Autodesk Inventor part; units mm, degrees
ref_plane "YZ Plane" through (0, 0, 0) normal (1, 0, 0) x (0, 1, 0)
ref_plane "XZ Plane" through (0, 0, 0) normal (0, 1, 0) x (-1, 0, 0)
ref_plane "XY Plane" through (0, 0, 0) normal (0, 0, 1) x (1, 0, 0)
sketch "Esquisse1" plane through (0, 0, 0) normal (0, 0, 1) x (1, 0, 0)
  line L0 (-12.5, -10) -> (12.5, -10)
  line L1 (12.5, -10) -> (12.5, 10)
  line L2 (12.5, 10) -> (-12.5, 10)
  line L3 (-12.5, 10) -> (-12.5, -10)
  line L4 (-12.5, -10) -> (12.5, 10) construction
  line L5 (12.5, -10) -> (-12.5, 10) construction
  point P0 (0, 0)
  dimension "d0" = 25
  dimension "d1" = 20
extrude "Extrusion1" add sketch "Esquisse1" along normal blind 7
sketch "Esquisse2" plane through (0, 0, 7) normal (0, 0, 1) x (1, 0, 0)
  line L0 (12.5, -10) -> (12.5, 10)
  line L1 (-12.5, 10) -> (-12.5, -10)
  line L2 (12.5, 10) -> (-12.5, 10)
  line L3 (-12.5, 10) -> (-12.5, 5)
  line L4 (-12.5, 5) -> (12.5, 5)
  line L5 (12.5, 5) -> (12.5, 10)
  point P0 (0, 0)
  point P1 (12.5, 5)
  dimension "d4" = 5
extrude "Extrusion2" add sketch "Esquisse2" along normal blind 3
sketch "Esquisse3" plane through (-12.5, 10, 0) normal (0, 1, 0) x (1, 0, 0)
  line L0 (25, 0) -> (25, -10)
  line L1 (25, -10) -> (24.1, -10)
  line L2 (24.1, -10) -> (24.1, -8)
  line L3 (24.1, -8) -> (25, -8)
  line L4 (25, -8) -> (25, -10)
  line L5 (24.1, -10) -> (21.56, -10)
  line L6 (25, -10) -> (0, -10)
  line L7 (21.56, -10) -> (16.1469, -10)
  line L8 (21.56, -10) -> (20.66, -10)
  line L9 (20.66, -10) -> (20.66, -8)
  line L10 (20.66, -8) -> (21.56, -8)
  line L11 (21.56, -8) -> (21.56, -10)
  line L12 (20.66, -10) -> (18.12, -10)
  line L13 (18.12, -10) -> (17.22, -10)
  line L14 (17.22, -10) -> (17.22, -8)
  line L15 (17.22, -8) -> (18.12, -8)
  line L16 (18.12, -8) -> (18.12, -10)
  line L17 (17.22, -10) -> (14.68, -10)
  line L18 (14.68, -10) -> (13.78, -10)
  line L19 (13.78, -10) -> (13.78, -8)
  line L20 (13.78, -8) -> (14.68, -8)
  line L21 (14.68, -8) -> (14.68, -10)
  line L22 (13.78, -10) -> (11.24, -10)
  line L23 (11.24, -10) -> (10.34, -10)
  line L24 (10.34, -10) -> (10.34, -8)
  line L25 (10.34, -8) -> (11.24, -8)
  line L26 (11.24, -8) -> (11.24, -10)
  line L27 (10.34, -10) -> (7.8, -10)
  line L28 (7.8, -10) -> (6.9, -10)
  line L29 (6.9, -10) -> (6.9, -8)
  line L30 (6.9, -8) -> (7.8, -8)
  line L31 (7.8, -8) -> (7.8, -10)
  line L32 (6.9, -10) -> (4.36, -10)
  line L33 (4.36, -10) -> (3.46, -10)
  line L34 (3.46, -10) -> (3.46, -8)
  line L35 (3.46, -8) -> (4.36, -8)
  line L36 (4.36, -8) -> (4.36, -10)
  line L37 (3.46, -10) -> (0.92, -10)
  line L38 (0.92, -10) -> (0.02, -10)
  line L39 (0.02, -8) -> (0.92, -8)
  line L40 (0.92, -8) -> (0.92, -10)
  line L41 (0, -10) -> (0, -8)
  line L42 (0, -8) -> (0.02, -8)
  point P0 (12.5, 0)
  point P1 (3.46, -10)
  point P2 (4.36, -10)
  point P3 (6.9, -10)
  point P4 (7.8, -10)
  dimension "d7" = 2.54
  dimension "d11" = 0.9
  dimension "d12" = 2
  dimension "d13" = 2.54
  dimension "d14" = 0.9
  dimension "d15" = 2
  dimension "d16" = 2.54
  dimension "d17" = 0.9
  dimension "d18" = 2
  dimension "d19" = 2.54
  dimension "d20" = 0.9
  dimension "d21" = 2
  dimension "d22" = 2.54
  dimension "d23" = 0.9
  dimension "d24" = 2
  dimension "d25" = 2.54
  dimension "d26" = 0.9
  dimension "d27" = 2
  dimension "d28" = 2.54
  dimension "d29" = 0.9
  dimension "d30" = 2
  dimension "d33" = 2
extrude "Extrusion3" add sketch "Esquisse3" along normal blind 4
sketch "Esquisse4" plane through (-12.5, 10, 0) normal (0, 1, 0) x (1, 0, 0)
  line L0 (25, -7) -> (25, -10)
  line L1 (25, -10) -> (24.1, -10)
  line L2 (0, -10) -> (25, -10)
  line L3 (24.1, -10) -> (21.56, -10)
  line L4 (21.56, -10) -> (21.56, -8)
  line L5 (21.56, -8) -> (24.1, -8)
  line L6 (24.1, -8) -> (24.1, -10)
  line L7 (21.56, -10) -> (20.66, -10)
  line L8 (20.66, -10) -> (18.12, -10)
  line L9 (18.12, -10) -> (18.12, -8)
  line L10 (18.12, -8) -> (20.66, -8)
  line L11 (20.66, -8) -> (20.66, -10)
  line L12 (18.12, -10) -> (17.22, -10)
  line L13 (17.22, -10) -> (14.68, -10)
  line L14 (14.68, -10) -> (14.68, -8)
  line L15 (14.68, -8) -> (17.22, -8)
  line L16 (17.22, -8) -> (17.22, -10)
  line L17 (14.68, -10) -> (13.78, -10)
  line L18 (13.78, -10) -> (11.24, -10)
  line L19 (11.24, -10) -> (11.24, -8)
  line L20 (11.24, -8) -> (13.78, -8)
  line L21 (13.78, -8) -> (13.78, -10)
  line L22 (11.24, -10) -> (10.34, -10)
  line L23 (10.34, -10) -> (7.8, -10)
  line L24 (7.8, -10) -> (7.8, -8)
  line L25 (7.8, -8) -> (10.34, -8)
  line L26 (10.34, -8) -> (10.34, -10)
  line L27 (7.8, -10) -> (6.9, -10)
  line L28 (6.9, -10) -> (4.36, -10)
  line L29 (4.36, -10) -> (4.36, -8)
  line L30 (4.36, -8) -> (6.9, -8)
  line L31 (6.9, -8) -> (6.9, -10)
  line L32 (4.36, -10) -> (3.46, -10)
  line L33 (3.46, -10) -> (0.92, -10)
  line L34 (0.92, -10) -> (0.92, -8)
  line L35 (0.92, -8) -> (3.46, -8)
  line L36 (3.46, -8) -> (3.46, -10)
  point P0 (12.5, 0)
  point P1 (3.46, -10)
  point P2 (4.36, -10)
  point P3 (6.9, -10)
  point P4 (7.8, -10)
  dimension "d36" = 0.9
  dimension "d37" = 2.54
  dimension "d38" = 2
  dimension "d39" = 0.9
  dimension "d40" = 2.54
  dimension "d41" = 2
  dimension "d42" = 0.9
  dimension "d43" = 2.54
  dimension "d44" = 2
  dimension "d45" = 0.9
  dimension "d46" = 2.54
  dimension "d47" = 2
  dimension "d48" = 0.9
  dimension "d49" = 2.54
  dimension "d50" = 2
  dimension "d51" = 0.9
  dimension "d52" = 2.54
  dimension "d53" = 2
  dimension "d54" = 0.9
  dimension "d55" = 2.54
  dimension "d56" = 2
extrude "Extrusion4" cut sketch "Esquisse4" along normal through all both and the other way through all
properties part number "Gyroscope MPU6050"
CAD build for the part. Positions are in the model's coordinates, mm. A direction names the side the tool comes from. Give positions to 0.01 mm unless a question says otherwise; leave off trailing zeros. Loops run counter-clockwise (first coordinate to the right, second up) from the corner with the lowest first, then second, coordinate; pieces in that order, holes last. Notation, with made-up numbers: M -18.75,88 L 21.25,88 A27 cw 21.25,116 Z; hole C 44,76 d11. An arc over 180 degrees is marked long. Write each question's results on one line, items separated by ' | '.
Q1. Probe probe 1 along Y at (x, z) = (-1.75, 7.25); probe 2 along Y at (x, z) = (11.25, 4); probe 3 along Z at (x, y) = (-8.5, -7). List the from-to ranges inside material, lowest first.
Geometry check:
probe 1: y = 5 to 10 | probe 2: y = -10 to 10 | probe 3: z = 0 to 7
Q2. Mould opens along X. For faces 4 (the face through (12.5, 2, 4)), 5 (the face through (-8.14, 9, 9)), 6 (the face through (12, 14, 9)) say: pulls with the +X half, pulls with the -X half, needs draft (parallel to the pull), parting line crosses it, or undercut.
Geometry check:
face 4: pulls with the +X half | face 5: undercut | face 6: needs draft
Q3. Flat gauge pins, fed straight in: P1, Ø1, axis at x = 12, y = 11.5, coming from the -Z side; P2, Ø0.8, axis at x = 7, y = 6.5, coming from the +Z side; P3, Ø1.5, axis at x = -8, y = -3.5, coming from the +Z side. Where does each tip first touch, or does it go through?
Geometry check:
P1: stops at z = 8 | P2: stops at z = 8 | P3: stops at z = 7
Q4. Band-saw the part on A-A on x = -1.75. Write the cut outline in (y, z).
Geometry check:
outline: M -10,0 L 10,0 L 10,8 L 14,8 L 14,10 L 5,10 L 5,7 L -10,7 Z
Q5. Band-saw the part on C-C on z = 4.75. Write the cut outline in (x, y), and give its area (3 significant figures).
Geometry check:
outline: M -12.5,-10 L 12.5,-10 L 12.5,10 L -12.5,10 Z | area: 500 mm²
Q6. Band-saw the part on D-D on x = 3.25. Write the cut outline in (y, z).
Geometry check:
outline: M -10,0 L 10,0 L 10,8 L 5,8 L 5,7 L -10,7 Z
Q7. Which spindle directions (+Z, -Z, +X, -X, +Y, -Y) get a long thin tool onto all of the face, cutting with end or side? Do faces 1 (the face through (-3, 7, 8)), 2 (the face through (5, 12, 8)), 3 (the face through (-8.6, 14, 9)). Say none if no direction does.
Geometry check:
face 1: +Z, +Y, -Y | face 2: -Z, +X, -X, +Y | face 3: +Z, -Z, +X, -X, +Y
